from build123d import *

# Parameters (mm, degrees)
SKETCH1_W           = 400
SKETCH1_H           = 500
BOSS_EXTRUDE1_DEPTH = 150
SKETCH2_W           = 400
SKETCH2_H           = 500
SKETCH2_W_2         = 355
SKETCH2_H_2         = 460
CUT_EXTRUDE1_DEPTH  = 17
SHELL1_T            = -1.5
SKETCH3_R           = 7.5
BOSS_EXTRUDE2_DEPTH = 14


with BuildPart() as part:
    # Sketch1 → Boss-Extrude1 (new body)
    with BuildSketch(Plane.XY):
        Rectangle(SKETCH1_W, SKETCH1_H)
    extrude(amount=BOSS_EXTRUDE1_DEPTH)

    # Sketch2 → Cut-Extrude1 (cut)
    with BuildSketch(Plane(origin=(0, 0, 0), x_dir=(-1, 0, 0), z_dir=(0, 0, -1))):
        Rectangle(SKETCH2_W, SKETCH2_H)
        Rectangle(SKETCH2_W_2, SKETCH2_H_2, mode=Mode.SUBTRACT)
    extrude(amount=-CUT_EXTRUDE1_DEPTH, mode=Mode.SUBTRACT)

    # Shell1
    shell1_openings = [part.faces().sort_by_distance(p)[0] for p in [
        (0, 0, 0),
    ]]
    offset(amount=SHELL1_T, openings=shell1_openings, kind=Kind.INTERSECTION)

    # Sketch3 → Boss-Extrude2 (add)
    with BuildSketch(Plane(origin=(0, 0, 148.5), x_dir=(-1, 0, 0), z_dir=(0, 0, -1))):
        with Locations(Location((-162.5, 202.5, 0), (0, 0, 180))):
            Circle(SKETCH3_R)
        with Locations(Location((162.5, 202.5, 0), (0, 0, 180))):
            Circle(SKETCH3_R)
        with Locations(Location((162.5, -202.5, 0), (0, 0, 180))):
            Circle(SKETCH3_R)
        with Locations(Location((-162.5, -202.5, 0), (0, 0, 180))):
            Circle(SKETCH3_R)
    extrude(amount=BOSS_EXTRUDE2_DEPTH)


solid = part.part
Could you check a few things on this model? Use its own coordinates, in mm. A direction names the side the tool comes from. Coordinates: 2 decimals unless noted, no trailing zeros. Order: outer loops, then holes, each group sorted by start corner. A loop starts at its lowest first (then second) coordinate and runs counter-clockwise, first axis right, second up. Notation, with made-up numbers: (57, 40.5) -> (70, 40.5) arc R14 ccw to (70, 67.5) -> close; hole circle Ø4 at (22.5, 20.25). An arc over 180 degrees is marked (long way). One line per item, written item: value. Start each with the question number.
1) Imagine slicing it at A-A on y = -202.5. List the corners of the cut face in (x, z) for me.
2) Imagine slicing it at D-D on y = 21. List the corners of the cut face in (x, z) for me, plus the area to 3 significant figures.
3) I'm going to push flat-ended pins straight in: pin 1 (13.5 mm diameter, centred on x = 86.5, z = 7.5, fed in from +Y); pin 2 (4.5 mm diameter, centred on x = 166, y = 200.5, fed in from -Z); pin 3 (6 mm diameter, centred on x = -88.5, y = 22.5, fed in from -Z). Where does each tip first touch, or does it pass through?
4) Imagine slicing it at B-B on z = 96.5. List the corners of the cut face in (x, y) for me, plus the area to 3 significant figures.
5) Which directions (+Z, -Z, +X, -X, +Y, -Y) give clear straight access to the entire face, cutting with the end or side of a thin tool? Please do faces 1 (the flat face through (200, -3, 83)), 2 (the flat face through (198.5, -3, 83)), 3 (the cylindrical face through (169.654, 200.247, 141.598)).
6) We'd pull the mould along X, two halves only. Please class faces 4 (the flat face through (-163, 202, 134.5)), 5 (the flat face through (-3, 248.5, 83)), 6 (the flat face through (177.5, -3, 8)), 7 (the flat face through (-177.5, -3, 8)): +X half, -X half, draft (parallel to the pull), parting line (faces both ways), or undercut.
7) If I drill on L1, parallel to X at y = 10, z = 97; L2, parallel to Y at x = 48, z = 106; L3, parallel to Z at x = -171.5, y = 187.5, over which ranges is the centre line in solid material (lowest first)? Write a range as [from, to].
8) Imagine slicing it at C-C on x = -124. List the corners of the cut face in (y, z) for me, plus the area to 3 significant figures.
Answer list:
1. outline: (-200, 17) -> (-177.5, 17) -> (-177.5, 0) -> (-176, 0) -> (-176, 18.5) -> (-198.5, 18.5) -> (-198.5, 148.5) -> (-170, 148.5) -> (-170, 134.5) -> (-155, 134.5) -> (-155, 148.5) -> (155, 148.5) -> (155, 134.5) -> (170, 134.5) -> (170, 148.5) -> (198.5, 148.5) -> (198.5, 18.5) -> (176, 18.5) -> (176, 0) -> (177.5, 0) -> (177.5, 17) -> (200, 17) -> (200, 150) -> (-200, 150) -> close
2. outline: (-200, 17) -> (-177.5, 17) -> (-177.5, 0) -> (-176, 0) -> (-176, 18.5) -> (-198.5, 18.5) -> (-198.5, 148.5) -> (198.5, 148.5) -> (198.5, 18.5) -> (176, 18.5) -> (176, 0) -> (177.5, 0) -> (177.5, 17) -> (200, 17) -> (200, 150) -> (-200, 150) -> close
2. area: 1,110 mm2
3. pin 1: stops at y = 230
3. pin 2: stops at z = 134.5
3. pin 3: stops at z = 148.5
4. outline: (-200, -250) -> (200, -250) -> (200, 250) -> (-200, 250) -> close; hole (-198.5, -248.5) -> (198.5, -248.5) -> (198.5, 248.5) -> (-198.5, 248.5) -> close
4. area: 2,690 mm2
5. face 1: +Z, -Z, +X, +Y, -Y
5. face 2: none
5. face 3: -Z
6. face 4: undercut
6. face 5: undercut
6. face 6: +X half
6. face 7: -X half
7. L1: x = [-200, -198.5], [198.5, 200]
7. L2: y = [-250, -248.5], [248.5, 250]
7. L3: z = [148.5, 150]
8. outline: (-250, 17) -> (-230, 17) -> (-230, 0) -> (-228.5, 0) -> (-228.5, 18.5) -> (-248.5, 18.5) -> (-248.5, 148.5) -> (248.5, 148.5) -> (248.5, 18.5) -> (228.5, 18.5) -> (228.5, 0) -> (230, 0) -> (230, 17) -> (250, 17) -> (250, 150) -> (-250, 150) -> close
8. area: 1,260 mm2
